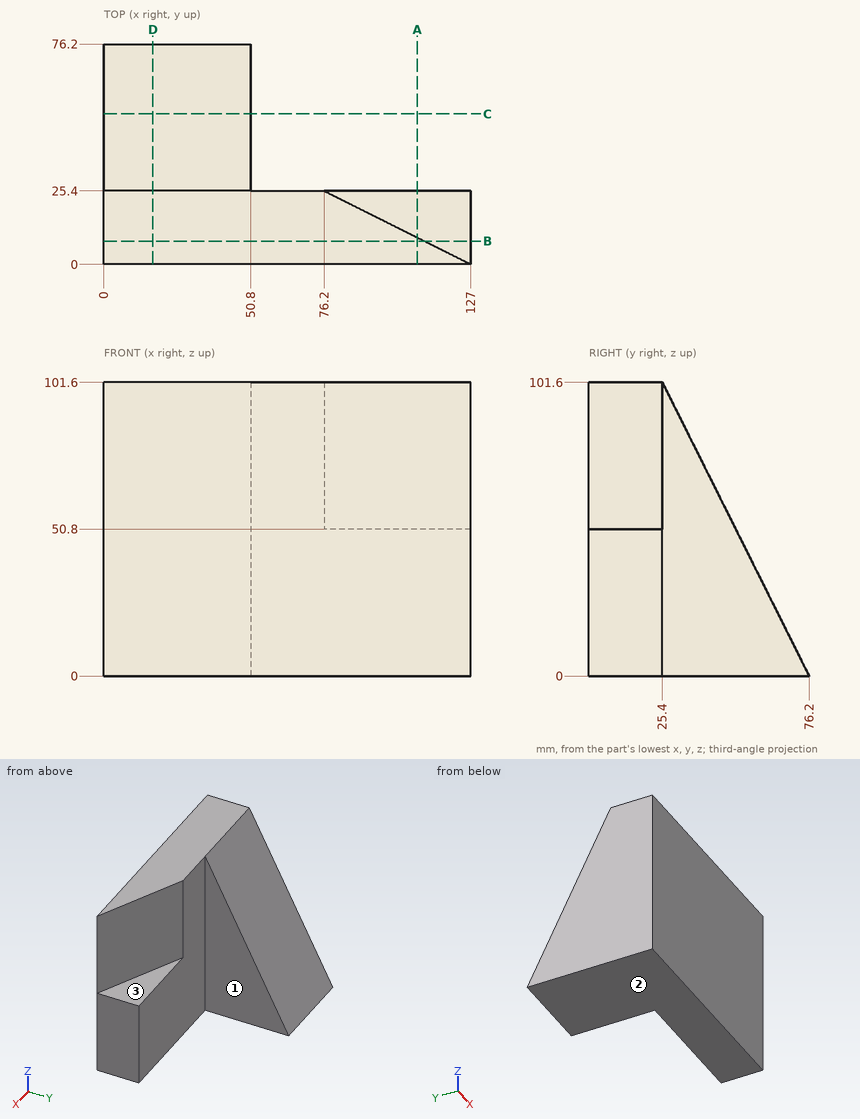
Verification items for this drawing (mm, ordinates from the low corner). A direction names the side the tool comes from. Coordinates: 2 decimals unless noted, no trailing zeros. Loops run counter-clockwise (first coordinate to the right, second up) from the corner with the lowest first, then second, coordinate; pieces in that order, holes last.
Item 1: Sectioned sample at A-A, the plane x = 108.5. Record the boundary of the cut face in (y, z), then the cut area to 3 significant figures.
Item 2: Thickness scan on line 1 (X direction, y = 26, z = 53); line 2 (Y direction, x = 99, z = 25.5). Record the ranges inside material, lowest first.
Item 3: Sectioned sample at C-C, the plane y = 52. Record the boundary of the cut face in (x, z).
Item 4: Sectioned sample at B-B, the plane y = 8. Record the boundary of the cut face in (x, z), then the cut area to 3 significant figures.
Item 5: Sectioned sample at D-D, the plane x = 17. Record the boundary of the cut face in (y, z).
Item 6: Access from +Z, -Z, +X, -X, +Y, -Y to the whole of each face (thin tool, end or side, straight path). Record for the marked faces 1, 2 and 3.
Item 7: Go/stop test with flat-tipped pins: pin 1 Ø12 at (y, z) = (63, 30) entering from -X; pin 2 Ø15 at (y, z) = (63, 40.5) entering from +X. Record where each tip stops, or that it passes through.
Check result:
1. outline: (0, 0) - (25.4, 0) - (25.4, 50.8) - (9.25, 50.8) - (9.25, 101.6) - (0, 101.6) - close
1. area: 1,760 mm2
2. line 1: x = 0 to 50.8
2. line 2: y = 0 to 25.4
3. outline: (0, 0) - (50.8, 0) - (50.8, 48.4) - (0, 48.4) - close
4. outline: (0, 0) - (127, 0) - (127, 50.8) - (111, 50.8) - (111, 101.6) - (0, 101.6) - close
4. area: 12,100 mm2
5. outline: (0, 0) - (76.2, 0) - (25.4, 101.6) - (0, 101.6) - close
6. face 1: +Z, -Z, +X, +Y
6. face 2: -Z, +X, -X, +Y, -Y
6. face 3: +Z, +X, +Y
7. pin 1: stops at x = 0
7. pin 2: stops at x = 50.8
